from build123d import *

# Parameters (mm, degrees)
SKETCH1_R               = 9.5
SKETCH1_R_2             = 7.6
BOSS_EXTRUDE1_DEPTH     = 5
SKETCH2_R               = 9.5
SKETCH2_R_2             = 1.31
BOSS_EXTRUDE2_DEPTH     = 2
SKETCH3_R               = 3.5
SKETCH3_R_2             = 1.6
BOSS_EXTRUDE3_DEPTH     = 15
CUT_EXTRUDE1_DEPTH      = 21.137030566
CUT_EXTRUDE1_DEPTH_BACK = 21.137030566
SKETCH3_3_R             = 1.31


with BuildPart() as part:
    # Sketch1 → Boss-Extrude1 (new body)
    with BuildSketch(Plane.XY):
        Circle(SKETCH1_R)
        Circle(SKETCH1_R_2, mode=Mode.SUBTRACT)
    extrude(amount=BOSS_EXTRUDE1_DEPTH)

    # Sketch2 → Boss-Extrude2 (add)
    with BuildSketch(Plane.XY.offset(5)):
        Circle(SKETCH2_R)
        Circle(SKETCH2_R_2, mode=Mode.SUBTRACT)
    extrude(amount=BOSS_EXTRUDE2_DEPTH)

    # Sketch3 → Boss-Extrude3 (add)
    with BuildSketch(Plane.XY.offset(7)):
        Circle(SKETCH3_R)
        Circle(SKETCH3_R_2, mode=Mode.SUBTRACT)
    extrude(amount=BOSS_EXTRUDE3_DEPTH)

    # Sketch3<3> → Cut-Extrude1 (cut, two sides: drawn at the far end of the back side and taken through both)
    with BuildSketch(Plane.XY.offset(7).offset(-CUT_EXTRUDE1_DEPTH_BACK)):
        with Locations((-5.5, 0)):
            Circle(SKETCH3_3_R)
        with Locations((5.5, 0)):
            Circle(SKETCH3_3_R)
    extrude(amount=CUT_EXTRUDE1_DEPTH + CUT_EXTRUDE1_DEPTH_BACK, mode=Mode.SUBTRACT)


solid = part.part
Geometry check sheet. Reference: the model listing, model coordinates, mm. A direction names the side the tool comes from. Give positions to 0.01 mm unless a question says otherwise; leave off trailing zeros. Loops run counter-clockwise (first coordinate to the right, second up) from the corner with the lowest first, then second, coordinate; pieces in that order, holes last.
(1) Thickness scan on L1, parallel to Y at x = 0, z = 1.9; L2, parallel to Z at x = -5.75, y = -6.5; L3, parallel to Z at x = 4.5, y = -5. Record the ranges inside material, lowest first.
From the geometry:
L1: y = -9.5 to -7.6, 7.6 to 9.5
L2: z = 0 to 7
L3: z = 5 to 7
(2) Section check C-C on z = 9.75. Record the cut outline in (x, y), then the cut area to 3 significant figures.
From the geometry:
outline: circle Ø7 at (0, 0); hole circle Ø3.2 at (0, 0)
area: 30.4 mm2
(3) Section check B-B on y = 7.25. Record the cut outline in (x, z), then the cut area to 3 significant figures.
From the geometry:
outline: (-6.14, 0) - (-2.28, 0) - (-2.28, 5) - (2.28, 5) - (2.28, 0) - (6.14, 0) - (6.14, 7) - (-6.14, 7) - close
area: 63.1 mm2
(4) Release check for a two-part mould opening along Y. For faces 1 (the cylindrical face through (4.38, -8.43, 3.45)), 2 (the flat face through (0, -2, 5)), 3 (the flat face through (1, -2, 22)), 4 (the cylindrical face through (-1.27, -0.97, 14.4)) record: released by +Y, released by -Y, zero draft, split by the parting line, or undercut.
From the geometry:
face 1: split by the parting line
face 2: undercut
face 3: zero draft
face 4: undercut
(5) Set-up check for faces 5 (the cylindrical face through (-4.25, 0.39, 5.99)), 6 (the cylindrical face through (3.233, -1.341, 14.395)), 7 (the cylindrical face through (-7.593, 0.334, 2.465)): record each of +Z, -Z, +X, -X, +Y, -Y from which the full face is reachable in a straight line by a thin tool's end or side.
From the geometry:
face 5: +Z, -Z
face 6: +Z
face 7: -Z
(6) Depth check by flat-ended pin: pin 1 Ø9.5 at (x, y) = (2.5, -3) entering from +Z; pin 2 Ø6 at (y, z) = (-1, 10.5) entering from -X; pin 3 Ø4 at (y, z) = (0, 15) entering from +X; pin 4 Ø1.6 at (x, y) = (0, 0) entering from -Z. Enter the tip coordinate at first touch or a pass-through.
From the geometry:
pin 1: stops at z = 22
pin 2: stops at x = -3.5
pin 3: stops at x = 3.5
pin 4: passes through
(7) Section check A-A on x = 0. Record the cut outline in (y, z).
From the geometry:
outline: (-9.5, 0) - (-7.6, 0) - (-7.6, 5) - (-1.31, 5) - (-1.31, 7) - (-1.6, 7) - (-1.6, 22) - (-3.5, 22) - (-3.5, 7) - (-9.5, 7) - close; (1.31, 5) - (7.6, 5) - (7.6, 0) - (9.5, 0) - (9.5, 7) - (3.5, 7) - (3.5, 22) - (1.6, 22) - (1.6, 7) - (1.31, 7) - close
(8) Section check D-D on x = -3. Record the cut outline in (y, z), then the cut area to 3 significant figures.
From the geometry:
outline: (-9.01, 0) - (-6.98, 0) - (-6.98, 5) - (6.98, 5) - (6.98, 0) - (9.01, 0) - (9.01, 7) - (1.8, 7) - (1.8, 22) - (-1.8, 22) - (-1.8, 7) - (-9.01, 7) - close
area: 110 mm2
